Work out the finished part from the listing and answer in its coordinate system (mm). Face numbers are marked on the shaded views. A direction names the side the tool comes from. Round coordinates to 2 decimals unless told otherwise and drop trailing zeros. Order: outer loops, then holes, each group sorted by start corner. A loop starts at its lowest first (then second) coordinate and runs counter-clockwise, first axis right, second up. Notation, with made-up numbers: (46.5, -40) - (57.5, -40) arc R19 cw to (57.5, -8) - close; hole circle Ø9 at (46.5, -1). An arc over 180 degrees is marked (long way). Answer in a Markdown table with one row per item.
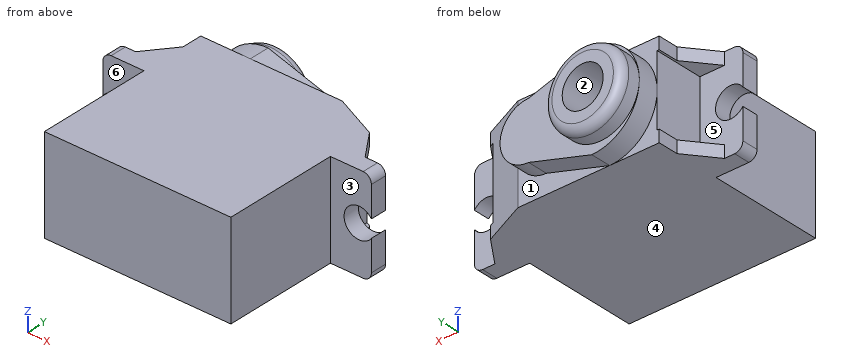
from build123d import *

# Parameters (mm, degrees)
BOSS_EXTRUDE1_DEPTH = 11.6
SKETCH2_R           = 1.833883236
CUT_EXTRUDE1_DEPTH  = 11.6
SKETCH3_W           = 28
SKETCH3_H           = 11.6
BOSS_EXTRUDE2_DEPTH = 6
SKETCH4_W           = 3
SKETCH4_H           = 8.622731964
CUT_EXTRUDE2_DEPTH  = 6
CUT_EXTRUDE3_DEPTH  = 12
BOSS_EXTRUDE3_DEPTH = 2.5
SKETCH7_R           = 4.75
BOSS_EXTRUDE4_DEPTH = 2.5
SKETCH8_R           = 2.5
CUT_EXTRUDE4_DEPTH  = 5
FILLET1_R           = 1


with BuildPart() as part:
    # Sketch1 → Boss-Extrude1 (new body)
    with BuildSketch(Plane.XY):
        Polygon((-9.992412141, 0), (12.757587859, 0), (12.757587859, 14), (17.757587859, 14), (17.757587859, 16), (-14.992412141, 16), (-14.992412141, 14), (-9.992412141, 14), align=None)
    extrude(amount=BOSS_EXTRUDE1_DEPTH)

    # Sketch2 → Cut-Extrude1 (cut)
    with BuildSketch(Plane(origin=(0, 16, 0), x_dir=(1, 0, 0), z_dir=(0, 1, 0))):
        with Locations((-13.492412141, -5.8)):
            Circle(SKETCH2_R)
        with Locations((16.257587859, -5.8)):
            Circle(SKETCH2_R)
    extrude(amount=-CUT_EXTRUDE1_DEPTH, mode=Mode.SUBTRACT)

    # Sketch3 → Boss-Extrude2 (add)
    with BuildSketch(Plane(origin=(0, 16, 0), x_dir=(1, 0, 0), z_dir=(0, 1, 0))):
        with Locations((1.257587859, -5.8)):
            Rectangle(SKETCH3_W, SKETCH3_H)
    extrude(amount=BOSS_EXTRUDE2_DEPTH)

    # Sketch4 → Cut-Extrude2 (cut)
    with BuildSketch(Plane(origin=(0, 22, 0), x_dir=(1, 0, 0), z_dir=(0, 1, 0))):
        with Locations((-11.242412141, -5.798634018)):
            Rectangle(SKETCH4_W, SKETCH4_H)
        with Locations((13.757587859, -5.798634018)):
            Rectangle(SKETCH4_W, SKETCH4_H)
    extrude(amount=-CUT_EXTRUDE2_DEPTH, mode=Mode.SUBTRACT)

    # Sketch5 → Cut-Extrude3 (cut)
    with BuildSketch(Plane.XY.offset(11.6)):
        Polygon((-9.992412141, 22), (-9.992412141, 19.5), (-12.742412141, 16), (-12.742412141, 22), align=None)
        Polygon((15.257587859, 16), (12.757587859, 19.5), (7.257587859, 22), (15.257587859, 22), align=None)
    extrude(amount=-CUT_EXTRUDE3_DEPTH, mode=Mode.SUBTRACT)

    # Sketch6 → Boss-Extrude3 (add)
    with BuildSketch(Plane(origin=(0, 22, 0), x_dir=(1, 0, 0), z_dir=(0, 1, 0))):
        with BuildLine():
            Line((-3.941512272, 0.001799738), (3.770704356, -2.312836319))
            ThreePointArc((3.770704356, -2.312836319), (7.257587859, -5.799719822), (3.770704356, -9.286603326))
            Line((3.770704356, -9.286603326), (-3.941512272, -11.6))
            ThreePointArc((-3.941512272, -11.6), (-9.742412141, -5.799100131), (-3.941512272, 0.001799738))
        make_face()
    extrude(amount=BOSS_EXTRUDE3_DEPTH)

    # Sketch7 → Boss-Extrude4 (add)
    with BuildSketch(Plane(origin=(0, 24.5, 0), x_dir=(1, 0, 0), z_dir=(0, 1, 0))):
        with Locations(Location((-4.992412141, -5.798937404, 0), (0, 0, 179.98128479))):
            Circle(SKETCH7_R)
    extrude(amount=BOSS_EXTRUDE4_DEPTH)

    # Sketch8 → Cut-Extrude4 (cut)
    with BuildSketch(Plane(origin=(0, 27, 0), x_dir=(1, 0, 0), z_dir=(0, 1, 0))):
        with Locations(Location((-4.992412141, -5.798937404, 0), (0, 0, 270))):
            Circle(SKETCH8_R)
    extrude(amount=-CUT_EXTRUDE4_DEPTH, mode=Mode.SUBTRACT)

    # Fillet1
    fillet1_edges = [part.edges().sort_by_distance(p)[0] for p in [
        (17.757587859, 15, 11.6),
        (-0.242412394, 27, 5.800488954),
        (-14.992412141, 15, 11.6),
        (-14.992412141, 15, 0),
        (17.757587859, 15, 0),
    ]]
    fillet(fillet1_edges, radius=FILLET1_R)


solid = part.part
1) The mould has two halves that part along Z. Classify the marked faces 4, 5 and 6: released by +Z, released by -Z, zero draft, split by the parting line, or undercut.
Filled in:
| item | result |
|---|---|
| face 4 | released by -Z |
| face 5 | undercut |
| face 6 | zero draft |
2) Which of the six approach directions +Z, -Z, +X, -X, +Y, -Y give full straight-line access (tool end or side, diameter ignored) to the marked faces 1, 2 and 3?
Filled in:
| item | result |
|---|---|
| face 1 | -Z, +X, +Y |
| face 2 | +Y |
| face 3 | +Z, -Z, +X, -Y |
3) Find the intervals of material crossed by probe 1 along Z at (x, y) = (2, 14.5); probe 2 along X at (y, z) = (14.7, 5.8); probe 3 along X at (y, z) = (13.5, 0.5), in increasing order. Write a range as from..to.
Filled in:
| item | result |
|---|---|
| probe 1 | z = 0..11.6 |
| probe 2 | x = -11.66..14.42 |
| probe 3 | x = -9.99..12.76 |
4) Find section A-A, the plane y = 14.75. Give the vertices of the cut face in (x, z), then the cut area to 3 significant figures.
Filled in:
| item | result |
|---|---|
| outline | (-14.99, 1) arc R1 ccw to (-13.99, 0) - (16.76, 0) arc R1 ccw to (17.76, 1) - (17.76, 4.74) arc R1.83 cw (long way) to (17.76, 6.86) - (17.76, 10.6) arc R1 ccw to (16.76, 11.6) - (-13.99, 11.6) arc R1 ccw to (-14.99, 10.6) - (-14.99, 6.86) arc R1.83 cw (long way) to (-14.99, 4.74) - close |
| area | 359 mm^2 |
5) Find section C-C, the plane x = 8. Give the vertices of the cut face in (y, z), then the cut area to 3 significant figures.
Filled in:
| item | result |
|---|---|
| outline | (0, 0) - (21.66, 0) - (21.66, 11.6) - (0, 11.6) - close |
| area | 251 mm^2 |
6) Each of these flat-tipped pins is pushed along its axis until it touches: pin 1 (1.5 mm diameter, centred on x = 0, z = 1.5, fed in from +Y); pin 2 (4 mm diameter, centred on x = -12.5, z = 4.5, fed in from -Y); pin 3 (1.7 mm diameter, centred on x = 15.5, z = 8, fed in from +Y). Where does it stop, or does it pass through?
Filled in:
| item | result |
|---|---|
| pin 1 | stops at y = 24.5 |
| pin 2 | stops at y = 14 |
| pin 3 | stops at y = 16 |
7) Find section B-B, the plane y = 24. Give the vertices of the cut face in (x, z).
Filled in:
| item | result |
|---|---|
| outline | (-3.94, 0) - (3.77, 2.31) arc R3.49 ccw to (3.77, 9.29) - (-3.94, 11.6) arc R5.8 ccw to start; hole circle Ø5 at (-4.99, 5.8) |
